Check sheet for the modelled part. Datum: model origin and axes. Units: mm. A direction names the side the tool comes from. Give positions to 0.01 mm unless a question says otherwise; leave off trailing zeros. Order: outer loops, then holes, each group sorted by start corner. A loop starts at its lowest first (then second) coordinate and runs counter-clockwise, first axis right, second up.
```python
from build123d import *

# Parameters (mm, degrees)
BOSS_EXTRUDE1_DEPTH         = 98.424999
BOSS_EXTRUDE1_DEPTH_BACK    = 98.424999
SKETCH3_W                   = 50.8
SKETCH3_H                   = 25.4
SKETCH3_W_2                 = 47.625
SKETCH3_H_2                 = 22.225
SKETCH4_R                   = 14.2875
CUT_EXTRUDE3_DEPTH          = 105.774999061
F_10_CLEARANCE_HOLE1_D      = 4.9784
F_20_0_161_DIAMETER_HOLE1_D = 4.0894
F_20_0_161_DIAMETER_HOLE2_D = 4.0894


with BuildPart() as part:
    # Sketch3 → Boss-Extrude1 (new, two sides: drawn at the far end of the back side and taken through both)
    with BuildSketch(Plane.XY.offset(-BOSS_EXTRUDE1_DEPTH_BACK)):
        Rectangle(SKETCH3_W, SKETCH3_H)
        Rectangle(SKETCH3_W_2, SKETCH3_H_2, mode=Mode.SUBTRACT)
    extrude(amount=BOSS_EXTRUDE1_DEPTH + BOSS_EXTRUDE1_DEPTH_BACK)

    # Sketch4 → Cut-Extrude3 (cut, through all)
    with BuildSketch(Plane.XZ.offset(12.7)):
        with Locations((0, 73.025)):
            Circle(SKETCH4_R)
        with Locations((0, -73.025)):
            Circle(SKETCH4_R)
    extrude(amount=-CUT_EXTRUDE3_DEPTH, mode=Mode.SUBTRACT)

    # #10 Clearance Hole1 (through all)
    with Locations(Plane(origin=(0, 12.7, 0), x_dir=(1, 0, 0), z_dir=(0, 1, 0))):
        with Locations((19.05, 38.099999492), (19.05, 92.074999492), (-19.05, 92.074999492), (-19.05, 38.099999492)):
            Hole(F_10_CLEARANCE_HOLE1_D / 2)

    # #20 (0.161) Diameter Hole1 (through all)
    with Locations(Plane(origin=(0, 12.7, 0), x_dir=(1, 0, 0), z_dir=(0, 1, 0))):
        with Locations((-12.751963692, -60.273036308), (12.751963691, -85.776963692)):
            Hole(F_20_0_161_DIAMETER_HOLE1_D / 2)

    # #20 (0.161) Diameter Hole2 (through all)
    with Locations(Plane(origin=(0, 12.7, 0), x_dir=(1, 0, 0), z_dir=(0, 1, 0))):
        with Locations((-15.293699364, 82.581564015), (15.293699363, 63.468435985)):
            Hole(F_20_0_161_DIAMETER_HOLE2_D / 2)


solid = part.part
```
(1) Cross-section at C-C on z = -38.1. Enter the section's corners in (x, y).
Response values:
outline: (-25.4, -12.7) - (-21.54, -12.7) - (-21.54, -11.11) - (-23.81, -11.11) - (-23.81, 11.11) - (-21.54, 11.11) - (-21.54, 12.7) - (-25.4, 12.7) - close; (-16.56, -12.7) - (16.56, -12.7) - (16.56, -11.11) - (-16.56, -11.11) - close; (-16.56, 11.11) - (16.56, 11.11) - (16.56, 12.7) - (-16.56, 12.7) - close; (21.54, -12.7) - (25.4, -12.7) - (25.4, 12.7) - (21.54, 12.7) - (21.54, 11.11) - (23.81, 11.11) - (23.81, -11.11) - (21.54, -11.11) - close
(2) Cross-section at D-D on z = -14. Enter the section's corners in (x, y), then the cut area to 3 significant figures.
Response values:
outline: (-25.4, -12.7) - (25.4, -12.7) - (25.4, 12.7) - (-25.4, 12.7) - close; hole (-23.81, -11.11) - (23.81, -11.11) - (23.81, 11.11) - (-23.81, 11.11) - close
area: 232 mm2
(3) Cross-section at B-B on x = 0. Enter the section's corners in (y, z) (1 decimal).
Response values:
outline: (-12.7, -98.4) - (-11.1, -98.4) - (-11.1, -87.3) - (-12.7, -87.3) - close; (-12.7, -58.7) - (-11.1, -58.7) - (-11.1, 58.7) - (-12.7, 58.7) - close; (-12.7, 87.3) - (-11.1, 87.3) - (-11.1, 98.4) - (-12.7, 98.4) - close; (11.1, -98.4) - (12.7, -98.4) - (12.7, -87.3) - (11.1, -87.3) - close; (11.1, -58.7) - (12.7, -58.7) - (12.7, 58.7) - (11.1, 58.7) - close; (11.1, 87.3) - (12.7, 87.3) - (12.7, 98.4) - (11.1, 98.4) - close
(4) Cross-section at A-A on y = 3.5. Enter the section's corners in (x, z) (1 decimal), then the cut area to 3 significant figures.
Response values:
outline: (-25.4, -98.4) - (-23.8, -98.4) - (-23.8, 98.4) - (-25.4, 98.4) - close; (23.8, -98.4) - (25.4, -98.4) - (25.4, 98.4) - (23.8, 98.4) - close
area: 625 mm2
(5) Set-up check for faces 1 (the face through (-13.85, 11.9, 58.55)), 2 (the face through (0, -11.112, -1)): record each of +Z, -Z, +X, -X, +Y, -Y from which the full face is reachable in a straight line by a thin tool's end or side.
Response values:
face 1: +Y, -Y
face 2: +Z, -Z
(6) Gauge pin test, flat end, axial feed: pin 1 Ø3.5 at (x, z) = (15.29, -63.47) entering from -Y. Record the tip position at first contact, or that the pin passes through.
Response values:
pin 1: passes through
(7) Material ranges on L1, parallel to Z at x = 0, y = 12.1 (1 decimal); L2, parallel to Y at x = -22, z = -31; L3, parallel to X at y = 0.5, z = 73, recorded low to high.
Response values:
L1: z = -98.4 to -87.3, -58.7 to 58.7, 87.3 to 98.4
L2: y = -12.7 to -11.11, 11.11 to 12.7
L3: x = -25.4 to -23.81, 23.81 to 25.4
(8) Release check for a two-part mould opening along Z. For faces 3 (the face through (13.02, 11.9, 83.75)), 4 (the face through (23.812, 0, -1)), 5 (the face through (0, -12, -98.425)) record: released by +Z, released by -Z, zero draft, split by the parting line, or undercut.
Response values:
face 3: undercut
face 4: zero draft
face 5: released by -Z
